Input: dimensioned drawing with shaded views. Units: mm. Origin: part minimum x, y, z. Coordinates: 2 decimals unless noted, no trailing zeros. Order: outer loops, then holes, each group sorted by start corner. A loop starts at its lowest first (then second) coordinate and runs counter-clockwise, first axis right, second up. Notation, with made-up numbers: (36.5, 25) - (52.5, 25) arc R21 cw to (52.5, 46) - close; hole circle Ø2 at (2, 83.5). An arc over 180 degrees is marked (long way). Answer as CSV lines item,"result". Start each with the question number.
Item 1: Section D-D (z = 23.25). Output: boundary loops of the cut face in (x, y).
Item 2: Section B-B (y = 12.25). Output: boundary loops of the cut face in (x, z) (3 decimals).
Item 3: First-contact query: pin 1 (2 mm diameter, centred on x = 17.5, y = 11, fed in from -Z); pin 2 (3 mm diameter, centred on x = 12.5, z = 19.5, fed in from -Y); pin 3 (6 mm diameter, centred on x = 16.5, y = 6.5, fed in from +Z); pin 4 (6 mm diameter, centred on y = 8, z = 23.5, fed in from +X). Flat tips, straight axial feed; report the tip coordinate or a pass-through.
Item 4: Material intervals for line 1 along Z through (x, y) = (15.25, 22); line 2 along Z through (x, y) = (11, 5.5); line 3 along X through (y, z) = (21.25, 8.5), sorted ascending.
Item 5: Section A-A (z = 11.5). Output: boundary loops of the cut face in (x, y), and give its area (3 significant figures).
Item 6: Section C-C (x = 24.75). Output: boundary loops of the cut face in (y, z), and give its area (3 significant figures).
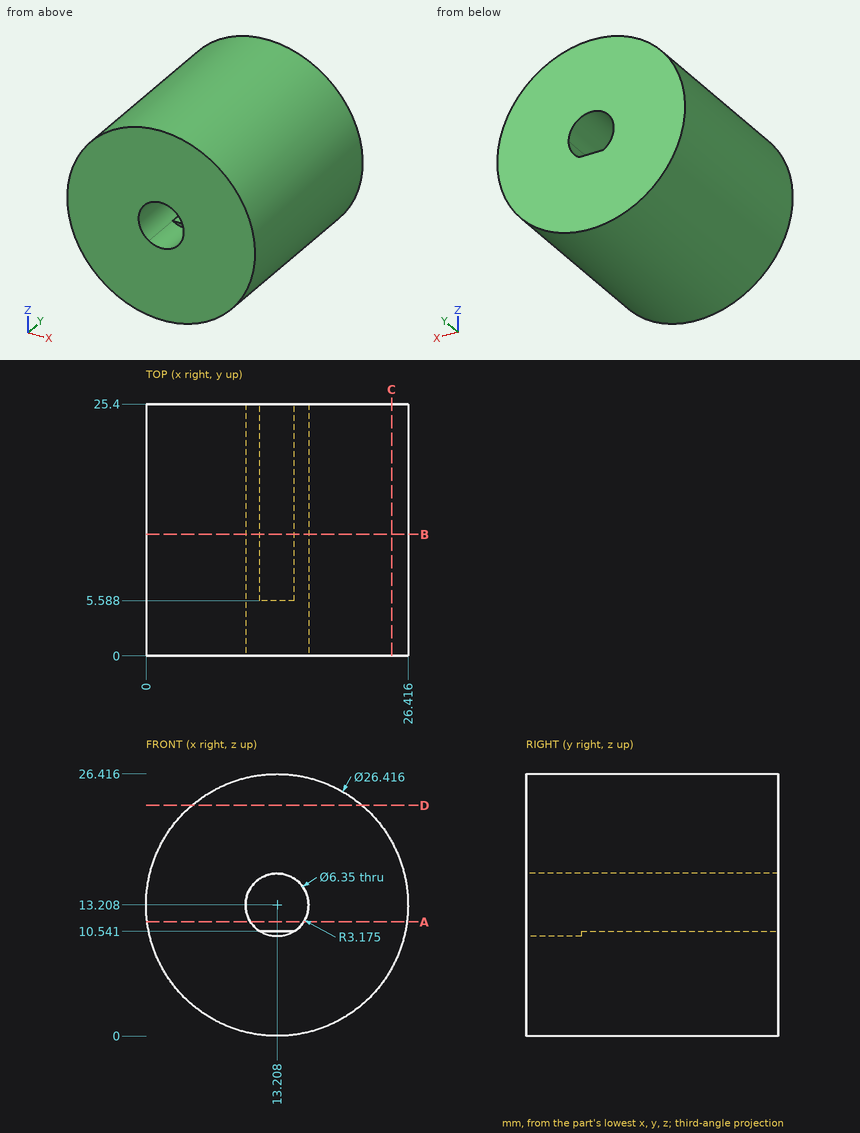
Determined:
1,outline,"(4.63, 0) - (21.79, 0) - (21.79, 25.4) - (4.63, 25.4) - close"
2,outline,"circle Ø26.416 at (13.208, 13.208); hole (11.485, 10.541) - (14.931, 10.541) arc R3.175 ccw (long way) to start"
3,pin 1,"stops at z = 0.42"
3,pin 2,"stops at y = 0"
3,pin 3,"stops at z = 26.41"
3,pin 4,"stops at x = 24.22"
4,line 1,"z = 0.16 to 10.78, 15.64 to 26.26"
4,line 2,"z = 0.19 to 10.93, 15.49 to 26.23"
4,line 3,"x = 0.87 to 25.55"
5,outline,"(0.11, 0) - (10.53, 0) - (10.53, 25.4) - (0.11, 25.4) - close; (15.88, 0) - (26.31, 0) - (26.31, 25.4) - (15.88, 25.4) - close"
5,area,"529 mm^2"
6,outline,"(0, 6.79) - (25.4, 6.79) - (25.4, 19.63) - (0, 19.63) - close"
6,area,"326 mm^2"
